Part model, mm, in its own coordinate system. A direction names the side the tool comes from. Round coordinates to 2 decimals unless told otherwise and drop trailing zeros. Write each loop counter-clockwise with the first axis right and the second up, starting at its lowest first coordinate (ties: lowest second). Pieces come first, ordered by that corner, then holes. Notation, with made-up numbers: M 23,31.5 L 64,31.5 A19 cw 64,67.5 Z; hole C 73,-30.5 d6. An arc over 180 degrees is marked long. Use one line per item in the form item = value. Start each with the question number.
Item 1: Flat gauge pins, fed straight in: pin 1 Ø1.6 at (x, z) = (-27.5, -18) entering from -Y; pin 2 Ø6.5 at (x, z) = (-1, -5) entering from +Y. Where does each tip first touch, or does it go through?
Item 2: Mould opens along Z. For faces 4 (the face through (1, 0.6, 7)), 5 (the face through (32.24, 0.79, -21.9)), 6 (the face through (-33.1, 1, 0)), 7 (the face through (30.578, 0.493, 17.638)) say: +Z half, -Z half, draft (parallel to the pull), parting line (faces both ways), or undercut.
Item 3: Cut at C-C, the plane z = 0.5. Give the cut face in (x, y), then the cut area to 3 significant figures.
Item 4: Cut at B-B, the plane x = -6.5. Give the cut face in (y, z), then the cut area to 3 significant figures.
Item 5: Cut at D-D, the plane y = 0.3. Give the cut face in (x, z).
Item 6: Cut at A-A, the plane z = -17.7. Give the cut face in (x, y), then the cut area to 3 significant figures.
Item 7: Probe L1, parallel to X at y = 1.55, z = 17.3; L2, parallel to Z at x = 15, y = 1.15; L3, parallel to Z at x = 11.5, y = 0.25. List the from-to ranges inside material, lowest first.
Item 8: Which spindle directions (+Z, -Z, +X, -X, +Y, -Y) get a long thin tool onto all of the face, cutting with end or side? Do faces 1 (the face through (12.93, 0.3, -7.2)), 2 (the face through (0, 1, 22.8)), 3 (the face through (-27.22, 0.49, -20.18)). Say none if no direction does.
from build123d import *

# Parameters (mm, degrees)
EXTRUDE_1_DEPTH        = 1.6
CUT_EXTRUDE_827_REACH  = 42.224
SKETCH_5_R             = 2.6
CUT_EXTRUDE_1317_DEPTH = 1
CUT_EXTRUDE_1453_REACH = 42.205
SKETCH_7_R             = 1.25
SKETCH_9_W             = 36
SKETCH_9_H             = 22
CUT_EXTRUDE_2013_DEPTH = 1


with BuildPart() as part:
    # 草图1 → 凸台-拉伸1 (new body)
    with BuildSketch(Plane(origin=(0, 0, 0), x_dir=(1, 0, 0), z_dir=(0, 1, 0))):
        with BuildLine():
            Line((-30.1, -22.8), (30.1, -22.8))
            ThreePointArc((30.1, -22.8), (32.221320344, -21.921320344), (33.1, -19.8))
            Line((33.1, -19.8), (33.1, 19.8))
            ThreePointArc((33.1, 19.8), (32.221320344, 21.921320344), (30.1, 22.8))
            Line((30.1, 22.8), (-30.1, 22.8))
            ThreePointArc((-30.1, 22.8), (-32.221320344, 21.921320344), (-33.1, 19.8))
            Line((-33.1, 19.8), (-33.1, -19.8))
            ThreePointArc((-33.1, -19.8), (-32.221320344, -21.921320344), (-30.1, -22.8))
        make_face()
    extrude(amount=EXTRUDE_1_DEPTH)

    # 草图3 → Cut-Extrude 827 (cut, up to next)
    with BuildSketch(Plane(origin=(0, 1.6, 0), x_dir=(1, 0, 0), z_dir=(0, 1, 0)), mode=Mode.PRIVATE) as cut_extrude_827_sk1:
        with BuildLine():
            Line((-8.5, -6.2), (11.5, -6.2))
            ThreePointArc((11.5, -6.2), (12.914213562, -5.614213562), (13.5, -4.2))
            Line((13.5, -4.2), (13.5, 5.8))
            ThreePointArc((13.5, 5.8), (12.914213562, 7.214213562), (11.5, 7.8))
            Line((11.5, 7.8), (-8.5, 7.8))
            ThreePointArc((-8.5, 7.8), (-9.914213562, 7.214213562), (-10.5, 5.8))
            Line((-10.5, 5.8), (-10.5, -4.2))
            ThreePointArc((-10.5, -4.2), (-9.914213562, -5.614213562), (-8.5, -6.2))
        make_face()
    cut_extrude_827_tool1 = extrude(cut_extrude_827_sk1.sketch, amount=-CUT_EXTRUDE_827_REACH, mode=Mode.PRIVATE) & part.part
    add(cut_extrude_827_tool1.solids().sort_by_distance((1.5, 1.6, -0.8))[0], mode=Mode.SUBTRACT)

    # 草图5 → Cut-Extrude 1317 (cut)
    with BuildSketch(Plane.XZ):
        with Locations(Location((-28, -17.7, 0), (0, 0, 270))):
            Circle(SKETCH_5_R)
        with Locations(Location((28, -17.7, 0), (0, 0, 270))):
            Circle(SKETCH_5_R)
        with Locations(Location((28, 17.3, 0), (0, 0, 270))):
            Circle(SKETCH_5_R)
        with Locations(Location((-28, 17.3, 0), (0, 0, 270))):
            Circle(SKETCH_5_R)
    extrude(amount=-CUT_EXTRUDE_1317_DEPTH, mode=Mode.SUBTRACT)

    # 草图7 → Cut-Extrude 1453 (cut, up to next)
    with BuildSketch(Plane.XZ.offset(-1), mode=Mode.PRIVATE) as cut_extrude_1453_sk1:
        with Locations(Location((-28, -17.7, 0), (0, 0, 270))):
            Circle(SKETCH_7_R)
    cut_extrude_1453_tool1 = extrude(cut_extrude_1453_sk1.sketch, amount=-CUT_EXTRUDE_1453_REACH, mode=Mode.PRIVATE) & part.part
    # 草图7 → Cut-Extrude 1453 (cut, up to next)
    with BuildSketch(Plane.XZ.offset(-1), mode=Mode.PRIVATE) as cut_extrude_1453_sk2:
        with Locations(Location((28, -17.7, 0), (0, 0, 270))):
            Circle(SKETCH_7_R)
    cut_extrude_1453_tool2 = extrude(cut_extrude_1453_sk2.sketch, amount=-CUT_EXTRUDE_1453_REACH, mode=Mode.PRIVATE) & part.part
    # 草图7 → Cut-Extrude 1453 (cut, up to next)
    with BuildSketch(Plane.XZ.offset(-1), mode=Mode.PRIVATE) as cut_extrude_1453_sk3:
        with Locations(Location((28, 17.3, 0), (0, 0, 270))):
            Circle(SKETCH_7_R)
    cut_extrude_1453_tool3 = extrude(cut_extrude_1453_sk3.sketch, amount=-CUT_EXTRUDE_1453_REACH, mode=Mode.PRIVATE) & part.part
    # 草图7 → Cut-Extrude 1453 (cut, up to next)
    with BuildSketch(Plane.XZ.offset(-1), mode=Mode.PRIVATE) as cut_extrude_1453_sk4:
        with Locations(Location((-28, 17.3, 0), (0, 0, 270))):
            Circle(SKETCH_7_R)
    cut_extrude_1453_tool4 = extrude(cut_extrude_1453_sk4.sketch, amount=-CUT_EXTRUDE_1453_REACH, mode=Mode.PRIVATE) & part.part
    add(cut_extrude_1453_tool1.solids().sort_by_distance((-28, 1, -17.7))[0], mode=Mode.SUBTRACT)
    add(cut_extrude_1453_tool2.solids().sort_by_distance((28, 1, -17.7))[0], mode=Mode.SUBTRACT)
    add(cut_extrude_1453_tool3.solids().sort_by_distance((28, 1, 17.3))[0], mode=Mode.SUBTRACT)
    add(cut_extrude_1453_tool4.solids().sort_by_distance((-28, 1, 17.3))[0], mode=Mode.SUBTRACT)

    # 草图9 → Cut-Extrude 2013 (cut)
    with BuildSketch(Plane(origin=(0, 1.6, 0), x_dir=(1, 0, 0), z_dir=(0, 1, 0))):
        with Locations((1.500900608, 0.362797629)):
            Rectangle(SKETCH_9_W, SKETCH_9_H)
    extrude(amount=-CUT_EXTRUDE_2013_DEPTH, mode=Mode.SUBTRACT)


solid = part.part
Model answer:
q1.pin_1 = 1
q1.pin_2 = 0.6
q2.face_4 = undercut
q2.face_5 = -Z half
q2.face_6 = draft
q2.face_7 = undercut
q3.outline = M -33.1,0 L -10.5,0 L -10.5,0.6 L -16.5,0.6 L -16.5,1.6 L -33.1,1.6 Z; M 13.5,0 L 33.1,0 L 33.1,1.6 L 19.5,1.6 L 19.5,0.6 L 13.5,0.6 Z
q3.area = 55.5 mm²
q4.outline = M 0,-22.8 L 1.6,-22.8 L 1.6,-11.36 L 0.6,-11.36 L 0.6,-7.8 L 0,-7.8 Z; M 0,6.2 L 0.6,6.2 L 0.6,10.64 L 1.6,10.64 L 1.6,22.8 L 0,22.8 Z
q4.area = 42.6 mm²
q5.outline = M -33.1,-19.8 A3 ccw -30.1,-22.8 L 30.1,-22.8 A3 ccw 33.1,-19.8 L 33.1,19.8 A3 ccw 30.1,22.8 L -30.1,22.8 A3 ccw -33.1,19.8 Z; hole C -28,-17.7 d5.2; hole C -28,17.3 d5.2; hole M -10.5,-5.8 A2 ccw -8.5,-7.8 L 11.5,-7.8 A2 ccw 13.5,-5.8 L 13.5,4.2 A2 ccw 11.5,6.2 L -8.5,6.2 A2 ccw -10.5,4.2 Z; hole C 28,-17.7 d5.2; hole C 28,17.3 d5.2
q6.outline = M -33.1,0 L -30.6,0 L -30.6,1 L -29.25,1 L -29.25,1.6 L -33.1,1.6 Z; M -26.75,1 L -25.4,1 L -25.4,0 L 25.4,0 L 25.4,1 L 26.75,1 L 26.75,1.6 L -26.75,1.6 Z; M 29.25,1 L 30.6,1 L 30.6,0 L 33.1,0 L 33.1,1.6 L 29.25,1.6 Z
q6.area = 92.5 mm²
q7.L1 = -33.1 to -29.25, -26.75 to 26.75, 29.25 to 33.1
q7.L2 = -22.8 to -11.36, 10.64 to 22.8
q7.L3 = -22.8 to -7.8, 6.2 to 22.8
q8.face_1 = +Y, -Y
q8.face_2 = +Z, +X, -X, +Y, -Y
q8.face_3 = -Y
